Geometry: final body of the model. Coordinates: model frame, mm. A direction names the side the tool comes from. Coordinates: 2 decimals unless noted, no trailing zeros. Loops run counter-clockwise (first coordinate to the right, second up) from the corner with the lowest first, then second, coordinate; pieces in that order, holes last. Notation, with made-up numbers: (3, 80) - (57, 80) arc R29 ccw to (57, 110) - close; hole circle Ø2 at (45, 86). An arc over 180 degrees is marked (long way). Put each result on its own line as item: value. Start each with the question number.
1) Reachability of faces 1 (the flat face through (14, 4, -4)), 2 (the cylindrical face through (7.368, 3.075, -4.01)) from +Z, -Z, +X, -X, +Y, -Y: full face, straight path, thin tool, end or side. Return the list, or none.
2) Section C-C on x = 24.5. Output: boundary loops of the cut face in (y, z), and give its area (3 significant figures).
3) Section B-B on x = 12. Output: boundary loops of the cut face in (y, z), and give its area (3 significant figures).
4) Section A-A on y = 0. Output: boundary loops of the cut face in (x, z).
5) Material intervals for line 1 along Y through (x, z) = (4, 0); line 2 along Z through (x, y) = (8, 0); line 3 along Z through (x, y) = (16.5, 16), sorted ascending. Write a range as from..to.
6) Draft query along Y for faces 3 (the flat face through (8.161, -20.486, -0.034)), 4 (the flat face through (7.9, 20.2, 0)), 5 (the cylindrical face through (32.2, -27.43, -0.03)), 6 (the flat face through (21, -19, 2.45)). Return one class per face: +Y half, -Y half, draft (parallel to the pull), parting line (faces both ways), or undercut.
7) Section D-D on y = -24.5. Output: boundary loops of the cut face in (x, z), and give its area (3 significant figures).
8) Contact query for flat-ended pins moving along their axis: pin 1 Ø5 at (x, z) = (30, -0.5) entering from -Y; pin 2 Ø7 at (x, y) = (14.5, -19.5) entering from -Z; pin 3 Ø7 at (x, y) = (19, -16) entering from +Z. Output: stop coordinate, or through.
Autodesk Inventor part; units mm, degrees
ref_plane "Work Plane1" through (76.6567, 0, 0) normal (0, 0, -1) x (1, 0, 0)
ref_plane "YZ Plane" through (0, 0, 0) normal (1, 0, 0) x (0, 1, 0)
ref_plane "XZ Plane" through (0, 0, 0) normal (0, 1, 0) x (-1, 0, 0)
sketch "Skizze1" plane through (0, 0, 0) normal (0, 0, 1) x (1, 0, 0)
  line L0 (0, 0) -> (14, 0)
  line L1 (0, 0) -> (0, 11.5)
  line L2 (14, 9.75) -> (14, 0)
  line L3 (0, 11.5) -> (16.0976, 29.2234)
  line L4 (14, 9.75) -> (25.9766, 12.8115)
  arc A0 (25.9766, 12.8115) -> (16.0976, 29.2234) centre (23.5, 22.5) ccw
  line L5 (14, 9.75) -> (0, 11.5)
  line L6 (14, 9.75) -> (0, 6.1712)
  dimension "d0" = 19.5
  dimension "d1" = 23.5
  dimension "d2" = 22.5
  dimension "d3" = 10
  dimension "d4" = 14
  dimension "d5" = 23
revolve "Körper" add sketch "Skizze1" angle 360 about axis through (0, 0, 0) along (1, 0, 0) contours L1 L6 L2 L0 | L1 L5 L6
extrude "Flügel1" add sketch "Skizze1" along normal mid plane 4.9 contours L1 L5 L6 | L5 L3 A0 L4
fillet "Rundung1" [suppressed]
mirror "Flügel2" about plane through (0, 0, 0) normal (0, 1, 0) of "Flügel1"
sketch "Skizze2" plane through (0, 0, 0) normal (1, 0, 0) x (0, 1, 0)
  line L0 (0, -14) -> (0, 14)
  line L1 (-14, 0) -> (14, 0)
  point P0 (0, 0)
hole "Gewinde" at (0, 0, 0) direction (1, 0, 0) diameter 10.106 end through all
chamfer "Fase1" distance 0.9472 angle 30 1 edges at (0, 0, -5.053) measured on face at (0, -9.1627, 0.203)
ref_plane "Work Plane1" through (76.6567, 0, 0) normal (0, 0, -1) x (1, 0, 0)
equation "\"d0\" = KOD2"
equation "\"d1\" = KOH1 - RR"
equation "\"d2\" = 0.5 * E0 - RR"
equation "\"d3\" = RR"
equation "\"d4\" = KOH"
equation "\"d5\" = KOD"
equation "\"d6\" = SW"
equation "\"d8\" = 0.333333 * SW"
equation "\"d9\" = -0.5 * GD1 + 0.5 * NND"
equation "\"d109\" = -0.5 * GD1 + 0.5 * NND"
equation "\"NND\" = 12"
equation "\"KOH\" = 14"
equation "\"KOH1\" = 33.5"
equation "\"SW\" = 4.9"
equation "\"KOD\" = 23"
equation "\"KOD2\" = 19.5"
equation "\"RR\" = 10"
equation "\"E0\" = 65"
equation "\"GUL\" = 0.541266 * PTC"
equation "\"BOR\" = 0"
equation "\"PTC\" = 1.75"
equation "\"THREADDIA\" = 12"
equation "\"TOA\" = 30deg"
equation "\"RR2\" = 6"
equation "\"SW1\" = 6.4"
equation "\"GAL\" = 0.541266 * PTC"
properties part number "DIN 315 - M12" material "Steel, Mild"
Answer block:
1. face 1: +Z, -Z, +X
1. face 2: +X, -X
2. outline: (-32.45, -2.45) - (-12.43, -2.45) - (-12.43, 2.45) - (-32.45, 2.45) - close; (12.43, -2.45) - (32.45, -2.45) - (32.45, 2.45) - (12.43, 2.45) - close
2. area: 196 mm²
3. outline: (-24.71, -2.45) - (-9.7, -2.45) arc R10 ccw to (9.7, -2.45) - (24.71, -2.45) - (24.71, 2.45) - (9.7, 2.45) arc R10 ccw to (-9.7, 2.45) - (-24.71, 2.45) - close; hole circle Ø10.11 at (0, 0)
3. area: 379 mm²
4. outline: (0, -11.5) - (14, -9.75) - (14, -5.05) - (0.55, -5.05) - (0, -6) - close; (0, 6) - (0.55, 5.05) - (14, 5.05) - (14, 9.75) - (0, 11.5) - close
5. line 1: y = -15.9..-5.05, 5.05..15.9
5. line 2: z = -10.5..-5.05, 5.05..10.5
5. line 3: z = -2.45..2.45
6. face 3: -Y half
6. face 4: +Y half
6. face 5: undercut
6. face 6: draft
7. outline: (11.81, -2.45) - (33.3, -2.45) - (33.3, 2.45) - (11.81, 2.45) - close
7. area: 105 mm²
8. pin 1: stops at y = -31.67
8. pin 2: stops at z = -2.45
8. pin 3: stops at z = 2.45
